```python
from build123d import *

# Parameters (mm, degrees)
F0_W     = 623
F0_H     = 810
F1_DEPTH = 22
F2_W     = 18
F2_H     = 30
F3_DEPTH = 623
F4_W     = 7
F4_H     = 810
F5_DEPTH = 4


with BuildPart() as f1:
    # F0 (on Front) → F1 (new body)
    with BuildSketch(Plane.XZ):
        Rectangle(F0_W, F0_H)
    extrude(amount=F1_DEPTH)

    # F2 (on face) → F3 (cut)
    with BuildSketch(Plane.YZ.offset(311.5)):
        with Locations((-13, 0)):
            Rectangle(F2_W, F2_H)
    extrude(amount=-F3_DEPTH, mode=Mode.SUBTRACT)

    # F4 (on face) → F5 (cut)
    with BuildSketch(Plane(origin=(0, 0, 0), x_dir=(-1, 0, 0), z_dir=(0, 1, 0))):
        with Locations((-308, 0)):
            Rectangle(F4_W, F4_H)
        with Locations((308, 0)):
            Rectangle(F4_W, F4_H)
    extrude(amount=-F5_DEPTH, mode=Mode.SUBTRACT)


solid = f1.part
```
Part model, mm, in its own coordinate system. A direction names the side the tool comes from. Round coordinates to 2 decimals unless told otherwise and drop trailing zeros. Write each loop counter-clockwise with the first axis right and the second up, starting at its lowest first coordinate (ties: lowest second). Pieces come first, ordered by that corner, then holes. Notation, with made-up numbers: M 75.5,71 L 117.5,71 A17 cw 117.5,82 Z; hole C 24,-21.5 d4. An arc over 180 degrees is marked long. Answer as CSV lines item,"result". Start each with the question number.
1) Drop flat-ended pins along their axis: pin 1 (7.5 mm diameter, centred on x = -309.5, z = 210.5, fed in from +Y); pin 2 (1.2 mm diameter, centred on y = -1, z = 0, fed in from -X). Give the stop position or say it passes through.
2) Which spindle directions (+Z, -Z, +X, -X, +Y, -Y) get a long thin tool onto all of the face, cutting with end or side? Do faces 1 (the face through (311.5, -13, 207)), 2 (the face through (4, -13, -15)). Say none if no direction does.
3) Band-saw the part on B-B (x = -77.5). List the corners of the cut face in (y, z), then the cut area to 3 significant figures.
4) Band-saw the part on A-A (y = -18). List the corners of the cut face in (x, z), then the cut area to 3 significant figures.
5) Drill centre lines: L1, parallel to Z at x = -69, y = -18; L2, parallel to Y at x = 159, z = -5.5; L3, parallel to X at y = -3, z = -235.5. Where is each one in solid material? Low to high.
6) Mould opens along Z. For faces 3 (the face through (-4, 0, 6)), 4 (the face through (-4, -11, 405)), 5 (the face through (4, -13, 15)), 6 (the face through (4, -4, 0)) say: +Z half, -Z half, draft (parallel to the pull), parting line (faces both ways), or undercut.
Worked out:
1,pin 1,"y = -4"
1,pin 2,"x = -304.5"
2,face 1,"+Z, -Z, +X, +Y, -Y"
2,face 2,"+X, -X, -Y"
3,outline,"M -22,-405 L 0,-405 L 0,405 L -22,405 L -22,15 L -4,15 L -4,-15 L -22,-15 Z"
3,area,"17,300 mm²"
4,outline,"M -311.5,-405 L 311.5,-405 L 311.5,-15 L -311.5,-15 Z; M -311.5,15 L 311.5,15 L 311.5,405 L -311.5,405 Z"
4,area,"486,000 mm²"
5,L1,"-405 to -15, 15 to 405"
5,L2,"-4 to 0"
5,L3,"-304.5 to 304.5"
6,face 3,"draft"
6,face 4,"+Z half"
6,face 5,"undercut"
6,face 6,"undercut"
